Input: part model. Units: mm. Frame: model coordinates. Face numbers are marked on the shaded views. Coordinates: 2 decimals unless noted, no trailing zeros. Order: outer loops, then holes, each group sorted by start corner. A loop starts at its lowest first (then second) coordinate and runs counter-clockwise, first axis right, second up. Notation, with made-up numbers: (23, -20.5) -> (76, -20.5) arc R12 ccw to (76, -9.5) -> close; hole circle Ø9 at (6.25, -6). An arc over 180 degrees is marked (long way). Use one line per item in the form item = value. Start each with the question number.
1) Section query A-A on x = -10. Output: boundary loops of the cut face in (y, z), then the cut area to 3 significant figures.
2) Draft query along X for the marked faces 1, 2 and 3. Return one class per face: pulls with the +X half, pulls with the -X half, needs draft (parallel to the pull), parting line crosses it, or undercut.
3) Section query D-D on x = 0. Output: boundary loops of the cut face in (y, z) (3 decimals), then the cut area to 3 significant figures.
4) Pin query (flat end, axial travel): pin 1 (2.5 mm diameter, centred on x = 0, y = 48.5, fed in from +Z); pin 2 (4.5 mm diameter, centred on y = 50.5, z = 0.5, fed in from -X); pin 3 (1.5 mm diameter, centred on x = 9.5, z = 1, fed in from -Y); pin 4 (1 mm diameter, centred on x = -4.5, y = 23.5, fed in from +Z). Return the tip coordinate at first contact, or that it passes through.
5) Ray query, line 1 along Z through (x, y) = (0, 28.5) (3 decimals); line 2 along X through (y, z) = (34.5, 10). Return the intervals inside material, ascending.
6) Section query C-C on z = 8.75. Output: boundary loops of the cut face in (x, y).
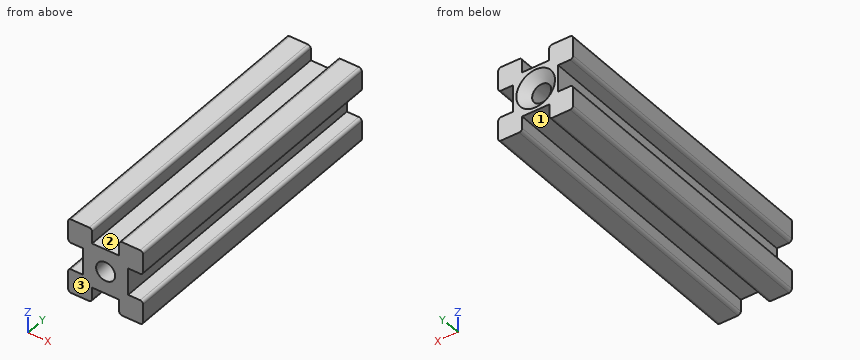
from build123d import *

# Parameters (mm, degrees)
SKETCH1_W                             = 25
SKETCH1_H                             = 25
BOSS_EXTRUDE1_DEPTH                   = 100
SKETCH2_W                             = 5
SKETCH2_H                             = 9
SKETCH2_W_2                           = 9
SKETCH2_H_2                           = 5
SKETCH2_W_3                           = 9.048888394
CUT_EXTRUDE1_DEPTH                    = 100
FILLET1_R                             = 1
F_1_4_0_25_DIAMETER_HOLE1_D           = 6.35
F_1_4_0_25_DIAMETER_HOLE1_CSINK_D     = 12.8778
F_1_4_0_25_DIAMETER_HOLE1_CSINK_ANGLE = 100


with BuildPart() as part:
    # Sketch1 → Boss-Extrude1 (new body)
    with BuildSketch(Plane(origin=(0, 0, 0), x_dir=(1, 0, 0), z_dir=(0, 1, 0))):
        Rectangle(SKETCH1_W, SKETCH1_H)
    extrude(amount=BOSS_EXTRUDE1_DEPTH)

    # Sketch2 → Cut-Extrude1 (cut)
    with BuildSketch(Plane(origin=(0, 100, 0), x_dir=(1, 0, 0), z_dir=(0, 1, 0))):
        with Locations((-10, 0)):
            Rectangle(SKETCH2_W, SKETCH2_H)
        with Locations((0, -10)):
            Rectangle(SKETCH2_W_2, SKETCH2_H_2)
        with Locations((-0.024444197, 10)):
            Rectangle(SKETCH2_W_3, SKETCH2_H_2)
        with Locations((10, 0)):
            Rectangle(SKETCH2_W, SKETCH2_H)
    extrude(amount=-CUT_EXTRUDE1_DEPTH, mode=Mode.SUBTRACT)

    # Fillet1
    fillet1_edges = [part.edges().sort_by_distance(p)[0] for p in [
        (-12.5, 50, 4.5),
        (-12.5, 50, -4.5),
        (-4.548888394, 50, -12.5),
        (4.5, 50, -12.5),
        (-4.5, 50, 12.5),
        (4.5, 50, 12.5),
        (12.5, 50, -4.5),
        (12.5, 50, 4.5),
        (12.5, 50, 12.5),
        (-12.5, 50, 12.5),
        (-12.5, 50, -12.5),
        (12.5, 50, -12.5),
    ]]
    fillet(fillet1_edges, radius=FILLET1_R)

    # 1/4 (0.25) Diameter Hole1 (through all)
    with Locations(Plane(origin=(0, 100, 0), x_dir=(1, 0, 0), z_dir=(0, 1, 0))):
        with Locations((0, 0)):
            CounterSinkHole(F_1_4_0_25_DIAMETER_HOLE1_D / 2, F_1_4_0_25_DIAMETER_HOLE1_CSINK_D / 2, counter_sink_angle=F_1_4_0_25_DIAMETER_HOLE1_CSINK_ANGLE)


solid = part.part
Answers below:
q1.outline = (0, -12.5) -> (100, -12.5) -> (100, -4.5) -> (0, -4.5) -> close; (0, 4.5) -> (100, 4.5) -> (100, 12.5) -> (0, 12.5) -> close
q1.area = 1,600 mm^2
q2.face_1 = undercut
q2.face_2 = undercut
q2.face_3 = needs draft
q3.outline = (0, -7.5) -> (100, -7.5) -> (100, -6.439) -> (97.261, -3.175) -> (0, -3.175) -> close; (0, 3.175) -> (97.261, 3.175) -> (100, 6.439) -> (100, 7.5) -> (0, 7.5) -> close
q3.area = 856 mm^2
q4.pin_1 = 7.5
q4.pin_2 = -7.5
q4.pin_3 = through
q4.pin_4 = 12.37
q5.line_1 = -7.5 to -3.175, 3.175 to 7.5
q5.line_2 = -12.5 to -4.5, 4.5 to 12.5
q6.outline = (-12.5, 0) -> (-4.5, 0) -> (-4.5, 100) -> (-12.5, 100) -> close; (4.5, 0) -> (12.5, 0) -> (12.5, 100) -> (4.5, 100) -> close
